Work out the finished part from the listing and answer in its coordinate system (mm). Face numbers are marked on the shaded views. A direction names the side the tool comes from. Round coordinates to 2 decimals unless told otherwise and drop trailing zeros. Write each loop counter-clockwise with the first axis right and the second up, starting at its lowest first coordinate (ties: lowest second). Pieces come first, ordered by that corner, then holes.
1. Find section A-A (x = -25). Write down the section's boundary in (y, z), and give its area (3 significant figures).
2. A tool of negligible diameter and unlimited length cuts with its end or side. For the marked faces 1, 2, 3 and 4, from which of +Z, -Z, +X, -X, +Y, -Y can it reach the whole face along a straight path? Write none if from no direction.
3. Find section D-D (z = 9.5). Write down the section's boundary in (x, y), and give its area (3 significant figures).
4. Find section B-B (z = -15). Write down the section's boundary in (x, y), and give its area (3 significant figures).
5. Determine the mould class of the marked faces 5, 6, 7 and 8 for opening direction Z: pulls with the +Z half, pulls with the -Z half, needs draft (parallel to the pull), parting line crosses it, or undercut.
6. Find section C-C (y = 2.15). Write down the section's boundary in (x, z).
7. Straight lines are drawn through the part: probe 1 along X at (y, z) = (4.6, -15); probe 2 along X at (y, z) = (4.55, 7); probe 3 along X at (y, z) = (4.5, -1). For each, find the intervals that lie inside material, in ascending order.
8. Flat-ended cylindrical pins translate along their axes: pin 1 Ø3 at (x, y) = (5.5, 5) entering from +Z; pin 2 Ø2 at (x, z) = (-12.5, 5) entering from +Y; pin 3 Ø3 at (x, y) = (-6.5, 2) entering from -Z; pin 4 Ø6 at (x, z) = (5.5, 2.5) entering from -Y. Find the tip coordinate at first contact, or state that the pin passes through.
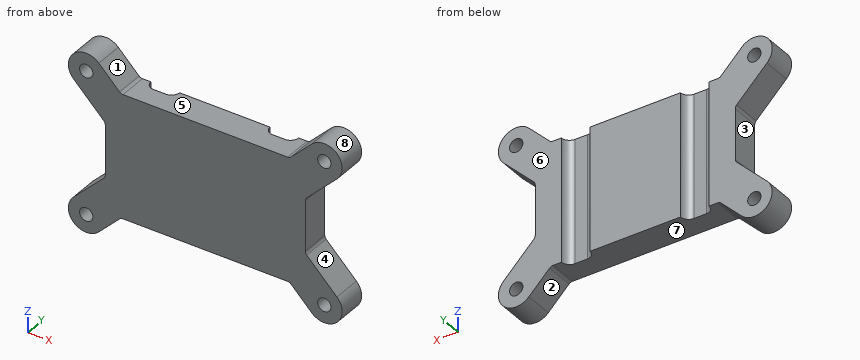
```python
from build123d import *

# Parameters (mm, degrees)
SKETCH1_R                 = 1.4
BASE_DEPTH                = 6
WIRE_GROOVES_DEPTH        = 44.250722537
F_1MM_SIDE_EDGE_FILLETS_R = 1


with BuildPart() as part:
    # Sketch1 → Base (new body)
    with BuildSketch(Plane(origin=(0, 0, 0), x_dir=(1, 0, 0), z_dir=(0, 1, 0))):
        with BuildLine():
            Line((-17.696699141, 13), (17.696699141, 13))
            Line((17.696699141, 13), (22.348349571, 17.651650429))
            ThreePointArc((22.348349571, 17.651650429), (27.651650429, 17.651650429), (27.651650429, 12.348349571))
            Line((27.651650429, 12.348349571), (21, 5.696699141))
            Line((21, 5.696699141), (21, -5.696699141))
            Line((21, -5.696699141), (27.651650429, -12.348349571))
            ThreePointArc((27.651650429, -12.348349571), (27.651650429, -17.651650429), (22.348349571, -17.651650429))
            Line((22.348349571, -17.651650429), (17.696699141, -13))
            Line((17.696699141, -13), (-17.696699141, -13))
            Line((-17.696699141, -13), (-22.348349571, -17.651650429))
            ThreePointArc((-22.348349571, -17.651650429), (-27.651650429, -17.651650429), (-27.651650429, -12.348349571))
            Line((-27.651650429, -12.348349571), (-21, -5.696699141))
            Line((-21, -5.696699141), (-21, 5.696699141))
            Line((-21, 5.696699141), (-27.651650429, 12.348349571))
            ThreePointArc((-27.651650429, 12.348349571), (-27.651650429, 17.651650429), (-22.348349571, 17.651650429))
            Line((-22.348349571, 17.651650429), (-17.696699141, 13))
        make_face()
        with Locations(Location((-25, 15, 0), (0, 0, 270))):
            Circle(SKETCH1_R, mode=Mode.SUBTRACT)
        with Locations(Location((-25, -15, 0), (0, 0, 270))):
            Circle(SKETCH1_R, mode=Mode.SUBTRACT)
        with Locations(Location((25, -15, 0), (0, 0, 270))):
            Circle(SKETCH1_R, mode=Mode.SUBTRACT)
        with Locations(Location((25, 15, 0), (0, 0, 270))):
            Circle(SKETCH1_R, mode=Mode.SUBTRACT)
    extrude(amount=BASE_DEPTH)

    # Sketch2 → Wire Grooves (cut, through all)
    with BuildSketch(Plane.XY.offset(13)):
        with BuildLine():
            Line((-15.496699141, 6), (-9.496699141, 6))
            ThreePointArc((-9.496699141, 6), (-9.994617613, 4.797918472), (-11.196699141, 4.3))
            Line((-11.196699141, 4.3), (-13.796699141, 4.3))
            ThreePointArc((-13.796699141, 4.3), (-14.998780669, 4.797918472), (-15.496699141, 6))
        make_face()
        with BuildLine():
            Line((9.503300859, 6), (15.503300859, 6))
            ThreePointArc((15.503300859, 6), (15.005382387, 4.797918472), (13.803300859, 4.3))
            Line((13.803300859, 4.3), (11.203300859, 4.3))
            ThreePointArc((11.203300859, 4.3), (10.001219331, 4.797918472), (9.503300859, 6))
        make_face()
    extrude(amount=-WIRE_GROOVES_DEPTH, mode=Mode.SUBTRACT)

    # 1mm Side Edge Fillets
    f_1mm_side_edge_fillets_edges = [part.edges().sort_by_distance(p)[0] for p in [
        (-17.696699141, 3, -13),
        (17.696699141, 3, -13),
        (21, 3, -5.696699141),
        (21, 3, 5.696699141),
        (17.696699141, 3, 13),
        (-17.696699141, 3, 13),
        (-21, 3, 5.696699141),
        (-21, 3, -5.696699141),
    ]]
    fillet(f_1mm_side_edge_fillets_edges, radius=F_1MM_SIDE_EDGE_FILLETS_R)


solid = part.part
```
Worked answers:
1. outline: (0, -18.75) - (6, -18.75) - (6, -16.4) - (0, -16.4) - close; (0, -13.6) - (6, -13.6) - (6, -9.7) - (0, -9.7) - close; (0, 9.7) - (6, 9.7) - (6, 13.6) - (0, 13.6) - close; (0, 16.4) - (6, 16.4) - (6, 18.75) - (0, 18.75) - close
1. area: 75.0 mm2
2. face 1: +Z, +Y, -Y
2. face 2: -Z, +Y, -Y
2. face 3: -X, +Y, -Y
2. face 4: +X, +Y, -Y
3. outline: (-24.8, 0) - (24.8, 0) - (24.8, 6) - (15.5, 6) arc R1.7 cw to (13.8, 4.3) - (11.2, 4.3) arc R1.7 cw to (9.5, 6) - (-9.5, 6) arc R1.7 cw to (-11.2, 4.3) - (-13.8, 4.3) arc R1.7 cw to (-15.5, 6) - (-24.8, 6) - close
3. area: 280 mm2
4. outline: (-28.75, 0) - (-26.4, 0) - (-26.4, 6) - (-28.75, 6) - close; (-23.6, 0) - (-19.7, 0) - (-19.7, 6) - (-23.6, 6) - close; (19.7, 0) - (23.6, 0) - (23.6, 6) - (19.7, 6) - close; (26.4, 0) - (28.75, 0) - (28.75, 6) - (26.4, 6) - close
4. area: 75.0 mm2
5. face 5: pulls with the +Z half
5. face 6: needs draft
5. face 7: pulls with the -Z half
5. face 8: undercut
6. outline: (-27.65, -12.35) arc R3.75 ccw to (-22.35, -17.65) - (-17.99, -13.29) arc R1 cw to (-17.28, -13) - (17.28, -13) arc R1 cw to (17.99, -13.29) - (22.35, -17.65) arc R3.75 ccw to (27.65, -12.35) - (21.29, -5.99) arc R1 cw to (21, -5.28) - (21, 5.28) arc R1 cw to (21.29, 5.99) - (27.65, 12.35) arc R3.75 ccw to (22.35, 17.65) - (17.99, 13.29) arc R1 cw to (17.28, 13) - (-17.28, 13) arc R1 cw to (-17.99, 13.29) - (-22.35, 17.65) arc R3.75 ccw to (-27.65, 12.35) - (-21.29, 5.99) arc R1 cw to (-21, 5.28) - (-21, -5.28) arc R1 cw to (-21.29, -5.99) - close; hole circle Ø2.8 at (-25, -15); hole circle Ø2.8 at (-25, 15); hole circle Ø2.8 at (25, -15); hole circle Ø2.8 at (25, 15)
7. probe 1: x = -28.75 to -26.4, -23.6 to -19.7, 19.7 to 23.6, 26.4 to 28.75
7. probe 2: x = -22.3 to -14.68, -10.31 to 10.32, 14.69 to 22.3
7. probe 3: x = -21 to -14.6, -10.4 to 10.4, 14.6 to 21
8. pin 1: stops at z = 13
8. pin 2: stops at y = 4.3
8. pin 3: stops at z = -13
8. pin 4: stops at y = 0
